Source: CAD feature listing. Evaluate the final solid. Frame: model axes, mm. A direction names the side the tool comes from. Give positions to 0.01 mm unless a question says otherwise; leave off trailing zeros. Loops run counter-clockwise (first coordinate to the right, second up) from the corner with the lowest first, then second, coordinate; pieces in that order, holes last. Notation, with made-up numbers: M 57.5,-20.75 L 91.5,-20.75 A22 cw 91.5,1.25 Z; hole C -13,31 d3. An arc over 180 degrees is marked long. Put each result on its own line as item: value.
Autodesk Inventor part; units mm, degrees
ref_plane "YZ Plane" through (0, 0, 0) normal (1, 0, 0) x (0, 1, 0)
ref_plane "XZ Plane" through (0, 0, 0) normal (0, 1, 0) x (-1, 0, 0)
ref_plane "XY Plane" through (0, 0, 0) normal (0, 0, 1) x (1, 0, 0)
sketch "Sketch1" plane through (0, 0, 0) normal (1, 0, 0) x (0, 1, 0)
  line L0 (22.225, 104.775) -> (136.525, 104.775)
  line L1 (136.525, 104.775) -> (136.525, -47.625)
  line L2 (136.525, -47.625) -> (22.225, -47.625)
  line L3 (22.225, -47.625) -> (22.225, 104.775)
  point P0 (0, 0)
  dimension "d0" = 114.3
  dimension "d1" = 152.4
extrude "Extrusion1" add sketch "Sketch1" along normal blind 7.62
sketch "Sketch2" plane through (7.62, 0, 0) normal (1, 0, 0) x (0, 0, -1)
  line L0 (-101.6, 133.35) -> (-84.1375, 133.35)
  line L1 (-84.1375, 133.35) -> (-84.1375, 122.2375)
  line L2 (-84.1375, 122.2375) -> (-101.6, 122.2375)
  line L3 (-101.6, 122.2375) -> (-101.6, 133.35)
  line L4 (-101.6, 26.9875) -> (-84.1375, 26.9875)
  line L5 (-84.1375, 26.9875) -> (-84.1375, 36.5125)
  line L6 (-84.1375, 36.5125) -> (-101.6, 36.5125)
  line L7 (-101.6, 36.5125) -> (-101.6, 26.9875)
  line L8 (44.45, 133.35) -> (28.575, 133.35)
  line L9 (28.575, 133.35) -> (28.575, 123.825)
  line L10 (28.575, 123.825) -> (44.45, 123.825)
  line L11 (44.45, 123.825) -> (44.45, 133.35)
  line L12 (44.45, 26.9875) -> (28.575, 26.9875)
  line L13 (28.575, 26.9875) -> (28.575, 36.5125)
  line L14 (28.575, 36.5125) -> (44.45, 36.5125)
  line L15 (44.45, 36.5125) -> (44.45, 26.9875)
  point P0 (0, 0)
extrude "Extrusion2" add sketch "Sketch2" along normal blind 88.265
sketch "Sketch3" plane through (0, 0, 0) normal (-1, 0, 0) x (0, 0, 1)
  line L0 (-47.625, 22.225) -> (-47.625, 136.525)
  line L1 (-47.625, 136.525) -> (104.775, 136.525)
  line L2 (-47.625, 22.225) -> (-39.6875, 22.225)
  line L3 (-39.6875, 22.225) -> (-39.6875, 136.525)
  line L4 (-39.6875, 136.525) -> (-47.625, 136.525)
  line L5 (-47.625, 136.525) -> (-47.625, 22.225)
  line L6 (104.775, 136.525) -> (104.775, 22.225)
  line L7 (-47.625, 136.525) -> (104.775, 136.525)
  line L8 (104.775, 136.525) -> (104.775, 128.5875)
  line L9 (-47.625, 128.5875) -> (-47.625, 136.525)
  line L10 (104.775, 22.225) -> (-47.625, 22.225)
  line L11 (104.775, 136.525) -> (96.8375, 136.525)
  line L12 (96.8375, 22.225) -> (104.775, 22.225)
  line L13 (104.775, 22.225) -> (104.775, 136.525)
  line L14 (-47.625, 22.225) -> (104.775, 22.225)
  line L15 (104.775, 22.225) -> (104.775, 30.1625)
  line L16 (104.775, 30.1625) -> (-47.625, 30.1625)
  line L17 (-47.625, 30.1625) -> (-47.625, 22.225)
  line L18 (-47.625, 136.525) -> (104.775, 136.525)
  line L19 (104.775, 136.525) -> (104.775, 128.5875)
  line L20 (104.775, 128.5875) -> (-47.625, 128.5875)
  line L21 (-47.625, 128.5875) -> (-47.625, 136.525)
  point P0 (0, 0)
extrude "Extrusion3" add sketch "Sketch3" along normal blind 17.78
sketch "Sketch4" plane through (7.62, 22.225, -47.625) normal (0, -1, 0) x (1, 0, 0)
  point P0 (-7.62, 47.625)
properties part number "TABLE NEW"
1. Section query B-B (y = 92). Output: boundary loops of the cut face in (x, z) (3 decimals), plus the area to 3 significant figures.
Found:
outline: M -17.78,-47.625 L 7.62,-47.625 L 7.62,104.775 L -17.78,104.775 Z
area: 3,870 mm^2
2. Section query A-A (x = 45). State how many separate pieces and enclosed holes the cut face has, plus the area to 3 significant figures.
Found:
separate pieces: 4
enclosed holes: 0
area: 663 mm^2
3. Contact query for flat-ended pins moving along their axis: P1, Ø7.5, axis at x = 61, y = 30, coming from the -Z side; P2, Ø4, axis at y = 45, z = 28, coming from the +X side; P3, Ø3, axis at x = 47.5, y = 31, coming from the +Z side. Output: stop coordinate, or through.
Found:
P1: z = -44.45
P2: x = 7.62
P3: z = 101.6
4. Material intervals for line 1 (Y direction, x = 34.5, z = 97); line 2 (X direction, y = 126, z = 80), sorted ascending. Write a range as from..to.
Found:
line 1: 26.99..36.51, 122.24..133.35
line 2: -17.78..7.62
5. Section query C-C (z = 68). Output: boundary loops of the cut face in (x, y) (3 decimals).
Found:
outline: M -17.78,22.225 L 7.62,22.225 L 7.62,136.525 L -17.78,136.525 Z
6. Draft query along Y for faces 1 (the flat face through (51, 122.238, 93)), 2 (the flat face through (51, 26.988, 93)), 3 (the flat face through (51, 129, -44.45)), 4 (the flat face through (51, 123.825, -36)). Return one class per face: pulls with the +Y half, pulls with the -Y half, needs draft (parallel to the pull), parting line crosses it, or undercut.
Found:
face 1: undercut
face 2: pulls with the -Y half
face 3: needs draft
face 4: undercut
7. Access query for faces 5 (the flat face through (51, 128, 101.6)), 6 (the flat face through (51, 32, -28.575)), 7 (the flat face through (51, 36.512, 93)). Directions: +Z, -Z, +X, -X, +Y, -Y. A direction counts if a zero-diameter tool reaches every point of the face in a straight line with its end or side. Return the directions, or none.
Found:
face 5: +Z, +X, +Y, -Y
face 6: +X, +Y, -Y
face 7: +Z, -Z, +X
